from build123d import *

# Parameters (mm, degrees)
SKETCH1_W           = 38.1
SKETCH1_H           = 76.2
BOSS_EXTRUDE1_DEPTH = 6.35
SKETCH8_W           = 19.05
SKETCH8_H           = 76.2
BOSS_EXTRUDE5_DEPTH = 6.35
SKETCH5_R           = 5.08
BOSS_EXTRUDE2_DEPTH = 10.414
SKETCH6_R           = 3.302
CUT_EXTRUDE3_DEPTH  = 57.429174157
SKETCH7_W           = 38.1
SKETCH7_H           = 12.7
BOSS_EXTRUDE4_DEPTH = 6.35
SKETCH9_R           = 2
CUT_EXTRUDE4_DEPTH  = 66.675579145
SKETCH10_W          = 12.954
SKETCH10_H          = 26.13
CUT_EXTRUDE5_DEPTH  = 2.54


with BuildPart() as part:
    # Sketch1 → Boss-Extrude1 (new body)
    with BuildSketch(Plane.XY):
        Rectangle(SKETCH1_W, SKETCH1_H)
    extrude(amount=BOSS_EXTRUDE1_DEPTH)

    # Sketch8 → Boss-Extrude5 (add)
    with BuildSketch(Plane.XY.offset(6.35)):
        with Locations((-28.575, 0)):
            Rectangle(SKETCH8_W, SKETCH8_H)
        with Locations((28.575, 0)):
            Rectangle(SKETCH8_W, SKETCH8_H)
    extrude(amount=-BOSS_EXTRUDE5_DEPTH)

    # Sketch5 → Boss-Extrude2 (add)
    with BuildSketch(Plane.XY.offset(6.35)):
        with Locations(Location((22.86, 25.4, 0), (0, 0, 180))):
            Circle(SKETCH5_R)
        with Locations(Location((-22.86, 25.4, 0), (0, 0, 180))):
            Circle(SKETCH5_R)
    boss_extrude2 = extrude(amount=BOSS_EXTRUDE2_DEPTH)

    # Sketch6 → Cut-Extrude3 (cut, through all)
    with BuildSketch(Plane.XY.offset(16.764)):
        with Locations((22.86, 25.4)):
            Circle(SKETCH6_R)
        with Locations(Location((-22.86, 25.4, 0), (0, 0, 180))):
            Circle(SKETCH6_R)
    cut_extrude3 = extrude(amount=-CUT_EXTRUDE3_DEPTH, mode=Mode.SUBTRACT)

    # Mirror1: Boss-Extrude2, Cut-Extrude3 across plane
    add(boss_extrude2.mirror(Plane.ZX))
    add(cut_extrude3.mirror(Plane.ZX), mode=Mode.SUBTRACT)

    # Sketch7 → Boss-Extrude4 (add)
    with BuildSketch(Plane.XY.offset(6.35)):
        with Locations((0, 44.45)):
            Rectangle(SKETCH7_W, SKETCH7_H)
    extrude(amount=-BOSS_EXTRUDE4_DEPTH)

    # Sketch9 → Cut-Extrude4 (cut, through all)
    with BuildSketch(Plane(origin=(0, 0, 0), x_dir=(-1, 0, 0), z_dir=(0, 0, -1))):
        with Locations((0, 29.21)):
            Circle(SKETCH9_R)
    extrude(amount=-CUT_EXTRUDE4_DEPTH, mode=Mode.SUBTRACT)

    # Sketch10 → Cut-Extrude5 (cut)
    with BuildSketch(Plane.XY):
        with Locations((0, 37.735)):
            Rectangle(SKETCH10_W, SKETCH10_H)
    extrude(amount=CUT_EXTRUDE5_DEPTH, mode=Mode.SUBTRACT)


solid = part.part
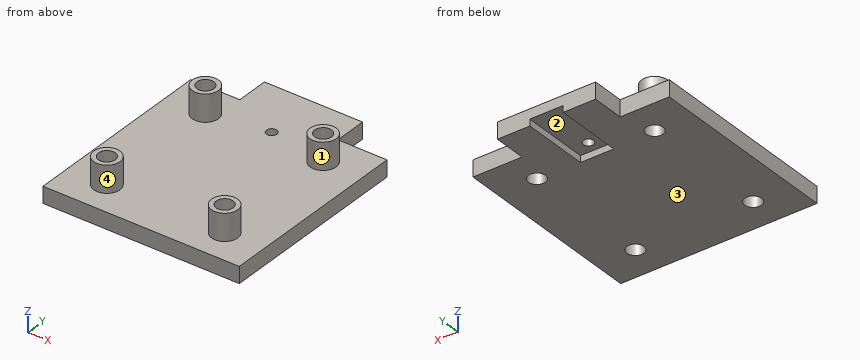
Build history of the part. All positions in model axes, mm. Face numbers are marked on the shaded views. A direction names the side the tool comes from. Round coordinates to 2 decimals unless told otherwise and drop trailing zeros. Write each loop counter-clockwise with the first axis right and the second up, starting at its lowest first coordinate (ties: lowest second). Pieces come first, ordered by that corner, then holes. Notation, with made-up numbers: M -5.75,47.25 L 18.25,47.25 A10 ccw 18.25,60.25 Z; hole C 48.5,-23 d11. An arc over 180 degrees is marked long. Answer in a Markdown table with one row per item.
1. Flat gauge pins, fed straight in: P1, Ø5, axis at x = -28, z = 4.5, coming from the +Y side; P2, Ø12, axis at x = -25, y = 6, coming from the +Z side; P3, Ø4, axis at x = -22.5, z = 14, coming from the -Y side; P4, Ø5.5, axis at x = -22.86, y = -25.4, coming from the +Z side. Where does each tip first touch, or does it go through?
Geometry check:
| item | result |
|---|---|
| P1 | y = 38.1 |
| P2 | z = 6.35 |
| P3 | y = -30.48 |
| P4 | through |
2. Saw through at B-B (x = 22.86). List the corners of the cut face in (y, z).
Geometry check:
| item | result |
|---|---|
| outline | M -38.1,0 L -28.7,0 L -28.7,16.76 L -30.48,16.76 L -30.48,6.35 L -38.1,6.35 Z; M -22.1,0 L 22.1,0 L 22.1,16.76 L 20.32,16.76 L 20.32,6.35 L -20.32,6.35 L -20.32,16.76 L -22.1,16.76 Z; M 28.7,0 L 38.1,0 L 38.1,6.35 L 30.48,6.35 L 30.48,16.76 L 28.7,16.76 Z |
3. Which spindle directions (+Z, -Z, +X, -X, +Y, -Y) get a long thin tool onto all of the face, cutting with end or side? Do the marked faces 1 and 2. Say none if no direction does.
Geometry check:
| item | result |
|---|---|
| face 1 | +Z |
| face 2 | -Z, +Y |
4. Mould opens along X. For the marked faces 3 and 4 say: +X half, -X half, draft (parallel to the pull), parting line (faces both ways), or undercut.
Geometry check:
| item | result |
|---|---|
| face 3 | draft |
| face 4 | undercut |
5. Saw through at A-A (z = 9.5). List the corners of the cut face in (x, y).
Geometry check:
| item | result |
|---|---|
| outline | C -22.86,-25.4 d10.16; C -22.86,25.4 d10.16; C 22.86,-25.4 d10.16; C 22.86,25.4 d10.16; hole C -22.86,-25.4 d6.6; hole C -22.86,25.4 d6.6; hole C 22.86,-25.4 d6.6; hole C 22.86,25.4 d6.6 |
6. Probe L1, parallel to Y at x = -22.86, z = 6; L2, parallel to Y at x = 20.5, z = 3.5; L3, parallel to X at y = -28, z = 13.5. List the from-to ranges inside material, lowest first. Write a range as [from, to].
Geometry check:
| item | result |
|---|---|
| L1 | [-38.1, -28.7], [-22.1, 22.1], [28.7, 38.1] |
| L2 | [-38.1, -27.71], [-23.09, 23.09], [27.71, 38.1] |
| L3 | [-27.22, -24.9], [-20.82, -18.5], [18.5, 20.82], [24.9, 27.22] |
7. Saw through at D-D (x = 0). List the corners of the cut face in (y, z).
Geometry check:
| item | result |
|---|---|
| outline | M -38.1,0 L 24.67,0 L 24.67,2.54 L 27.21,2.54 L 27.21,6.35 L -38.1,6.35 Z; M 31.21,2.54 L 50.8,2.54 L 50.8,6.35 L 31.21,6.35 Z |
8. Saw through at C-C (y = -25.4). List the corners of the cut face in (x, z), and give its area (3 significant figures).
Geometry check:
| item | result |
|---|---|
| outline | M -38.1,0 L -26.16,0 L -26.16,16.76 L -27.94,16.76 L -27.94,6.35 L -38.1,6.35 Z; M -19.56,0 L 19.56,0 L 19.56,16.76 L 17.78,16.76 L 17.78,6.35 L -17.78,6.35 L -17.78,16.76 L -19.56,16.76 Z; M 26.16,0 L 38.1,0 L 38.1,6.35 L 27.94,6.35 L 27.94,16.76 L 26.16,16.76 Z |
| area | 474 mm2 |
